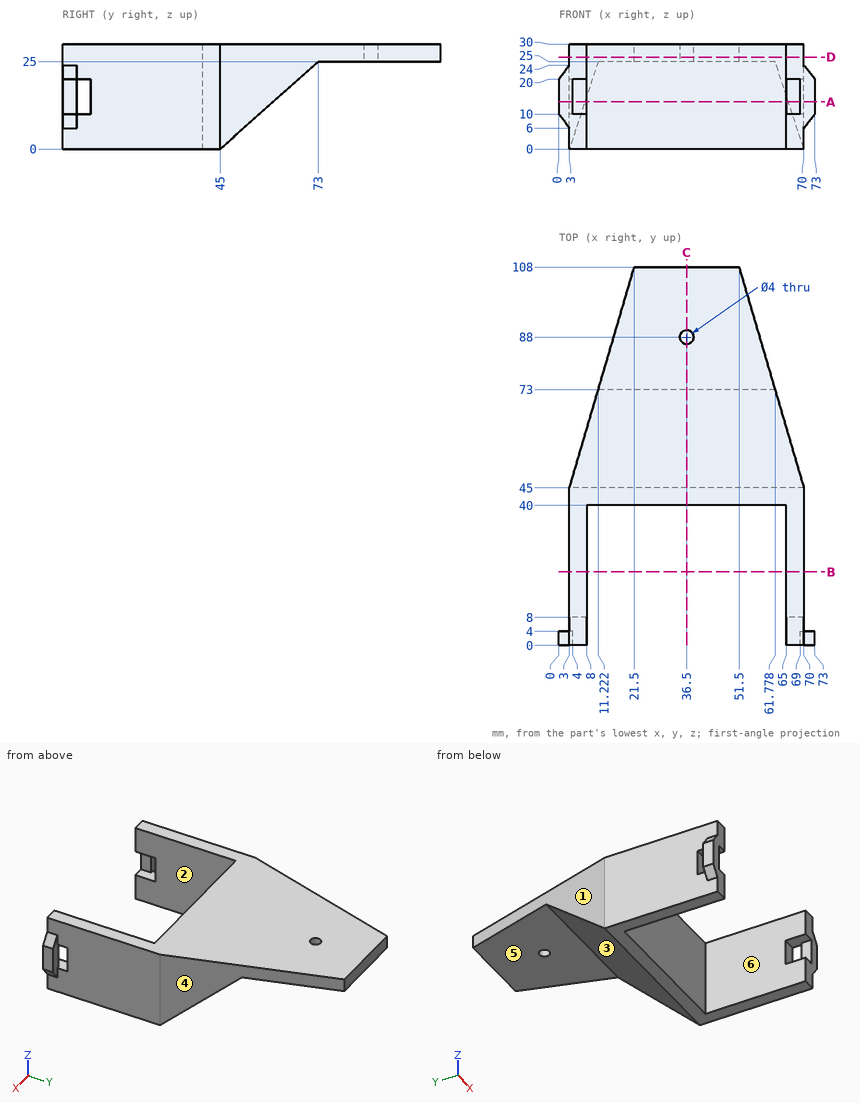
Geometry check sheet. Reference: drawing and pictorial views, mm from the part's lowest x, y, z. A direction names the side the tool comes from. Give positions to 0.01 mm unless a question says otherwise; leave off trailing zeros. Order: outer loops, then holes, each group sorted by start corner. A loop starts at its lowest first (then second) coordinate and runs counter-clockwise, first axis right, second up. Notation, with made-up numbers: M 15.5,6 L 51.5,6 A35 ccw 51.5,43 Z; hole C 77.5,-19.75 d3. An arc over 180 degrees is marked long. Answer in a Markdown table with one row per item. Add a question column.
Q1. Sectioned sample at A-A, the plane z = 13.5. Record the boundary of the cut face in (x, y), and give its area (3 significant figures).
Q2. Thickness scan on L1, parallel to Y at x = 36.5, z = 26.9; L2, parallel to X at y = 13, z = 17.75; L3, parallel to X at y = 42, z = 14.25. Record the ranges inside material, lowest first.
Q3. Gauge pin test, flat ends, axial feed: pin 1 Ø2 at (x, z) = (15, 21) entering from +Y; pin 2 Ø8 at (x, y) = (31, 97) entering from -Z; pin 3 Ø1.5 at (x, z) = (48, 17.5) entering from +Y. Record the tip position at first contact, or that the pin passes through.
Q4. Release check for a two-part mould opening along X. For the marked faces 1, 2 and 3 record: released by +X, released by -X, zero draft, split by the parting line, or undercut.
Q5. Sectioned sample at D-D, the plane z = 26.25. Record the boundary of the cut face in (x, y).
Q6. Access from +Z, -Z, +X, -X, +Y, -Y to the whole of each face (thin tool, end or side, straight path). Record for the marked faces 4, 5 and 6.
Q7. Sectioned sample at C-C, the plane x = 36.5. Record the boundary of the cut face in (y, z).
Q8. Sectioned sample at B-B, the plane y = 21. Record the boundary of the cut face in (x, z), and give its area (3 significant figures).
Verdict:
| question | item | result |
|---|---|---|
| 1 | outline | M 0,0 L 4,0 L 4,4 L 0,4 Z; M 3,8 L 8,8 L 8,40 L 65,40 L 65,8 L 70,8 L 70,45 L 65.56,60.12 L 7.44,60.12 L 3,45 Z; M 69,0 L 73,0 L 73,4 L 69,4 Z |
| 1 | area | 1,630 mm² |
| 2 | L1 | 40 to 86, 90 to 108 |
| 2 | L2 | 3 to 8, 65 to 70 |
| 2 | L3 | 3 to 70 |
| 3 | pin 1 | y = 69.64 |
| 3 | pin 2 | z = 25 |
| 3 | pin 3 | y = 65.44 |
| 4 | face 1 | released by -X |
| 4 | face 2 | undercut |
| 4 | face 3 | zero draft |
| 5 | outline | M 3,0 L 8,0 L 8,40 L 65,40 L 65,0 L 70,0 L 70,45 L 51.5,108 L 21.5,108 L 3,45 Z; hole C 36.5,88 d4 |
| 6 | face 4 | +Z, -Z, +X, +Y |
| 6 | face 5 | -Z, +X, -X, +Y |
| 6 | face 6 | +Z, -Z, -Y |
| 7 | outline | M 40,0 L 45,0 L 73,25 L 86,25 L 86,30 L 40,30 Z; M 90,25 L 108,25 L 108,30 L 90,30 Z |
| 8 | outline | M 3,0 L 8,0 L 8,30 L 3,30 Z; M 65,0 L 70,0 L 70,30 L 65,30 Z |
| 8 | area | 300 mm² |
